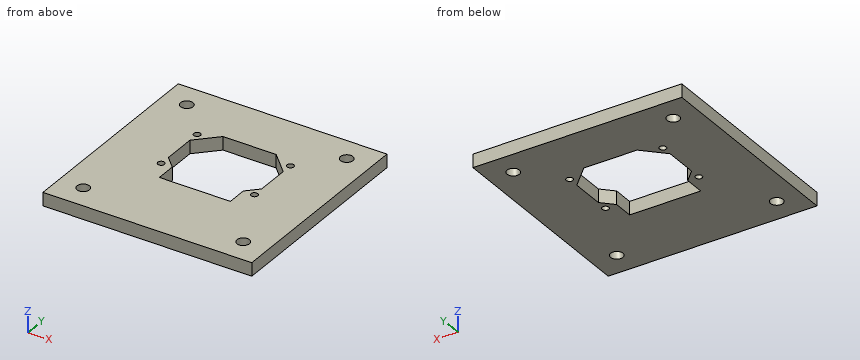
Autodesk Inventor part; units mm, degrees
ref_plane "YZ Plane" through (0, 0, 0) normal (1, 0, 0) x (0, 1, 0)
ref_plane "XZ Plane" through (0, 0, 0) normal (0, 1, 0) x (-1, 0, 0)
ref_plane "XY Plane" through (0, 0, 0) normal (0, 0, 1) x (1, 0, 0)
sketch "Sketch1" plane through (0, 0, 0) normal (0, 0, 1) x (1, 0, 0)
  circle A0 centre (-10.5, 10) radius 0.75
  circle A1 centre (-10.5, -2.5) radius 0.75
  circle A2 centre (10.5, 10) radius 0.75
  circle A3 centre (10.5, -2.5) radius 0.75
  line L0 (6, 12) -> (10.5, 7.5)
  line L1 (10.5, 7.5) -> (10.5, 0)
  line L2 (0, 15.2771) -> (0, -20.9272) construction
  line L3 (10.5, 0) -> (8, -2.5)
  line L4 (8, -2.5) -> (8, -7)
  line L5 (-6, 12) -> (-10.5, 7.5)
  line L6 (-10.5, 7.5) -> (-10.5, 0)
  line L7 (-10.5, 0) -> (-8, -2.5)
  line L8 (-8, -2.5) -> (-8, -7)
  line L9 (8, -7) -> (-8, -7)
  line L10 (23.5, 23.5) -> (23.5, -23.5)
  line L11 (23.5, -23.5) -> (-23.5, -23.5)
  line L12 (-23.5, -23.5) -> (-23.5, 23.5)
  line L13 (-23.5, 23.5) -> (23.5, 23.5)
  line L14 (6, 12) -> (-6, 12)
  line L15 (12.5, 12.5) -> (12.5, -12.5) construction
  line L16 (-12.5, -12.5) -> (-12.5, 12.5) construction
  line L17 (12.5, -12.5) -> (23.5, -23.5) construction
  line L18 (12.5, 12.5) -> (23.5, 23.5) construction
  line L19 (-12.5, 12.5) -> (-23.5, 23.5) construction
  line L20 (-12.5, -12.5) -> (-23.5, -23.5) construction
  circle A4 centre (18, -18) radius 1.4
  circle A5 centre (18, 18) radius 1.4
  circle A6 centre (-18, 18) radius 1.4
  circle A7 centre (-18, -18) radius 1.4
  line L21 (12.5, 12.5) -> (-12.5, -12.5) construction
  line L22 (12.5, -12.5) -> (-12.5, 12.5) construction
  point P0 (0, 0)
  point P1 (0, 0)
  point P2 (0, 0)
  point P3 (-8.25, 9.75)
  point P4 (0, 0)
  point P5 (0, 0)
  dimension "d2" = 1.5
  dimension "d5" = 1.5
  dimension "d8" = 1.5
  dimension "d11" = 1.5
  dimension "d48" = 2.8
  dimension "d49" = 2.8
  dimension "d50" = 2.8
  dimension "d51" = 2.8
  dimension "d63" = 15.5564
  dimension "d64" = 7.7782
  dimension "d66" = 7.7782
  dimension "d67" = 7.7782
  dimension "d68" = 47
extrude "Extrusion1" add sketch "Sketch1" along normal blind 3
equation "\"d64\" = 0.5 * d63"
equation "\"d66\" = d64"
equation "\"d67\" = d64"
properties part number "Camera-Holder_Mount"
Build history of the part. All positions in model axes, mm. Coordinates: 2 decimals unless noted, no trailing zeros. Order: outer loops, then holes, each group sorted by start corner. A loop starts at its lowest first (then second) coordinate and runs counter-clockwise, first axis right, second up. Notation, with made-up numbers: (-16.5, 71) - (34.5, 71) arc R22 cw to (34.5, 94) - close; hole circle Ø2 at (50.25, 53). An arc over 180 degrees is marked (long way). Put each result on its own line as item: value.
1. Drop a flat-ended pin along its axis: P1, Ø0.9, axis at x = -10.5, y = -2.5, coming from the -Z side. Give the stop position or say it passes through.
Answer sheet:
P1: passes through
2. Saw through at A-A (y = -18). Write the cut outline in (x, z), and give its area (3 significant figures).
Answer sheet:
outline: (-23.5, 0) - (-19.4, 0) - (-19.4, 3) - (-23.5, 3) - close; (-16.6, 0) - (16.6, 0) - (16.6, 3) - (-16.6, 3) - close; (19.4, 0) - (23.5, 0) - (23.5, 3) - (19.4, 3) - close
area: 124 mm^2
3. Probe line 1 along Y through (x, z) = (18, 2.2); line 2 along Y through (x, z) = (4.5, 0.85); line 3 along X through (y, z) = (-18.5, 2). List the from-to ranges inside material, lowest first. Write a range as [from, to].
Answer sheet:
line 1: y = [-23.5, -19.4], [-16.6, 16.6], [19.4, 23.5]
line 2: y = [-23.5, -7], [12, 23.5]
line 3: x = [-23.5, -19.31], [-16.69, 16.69], [19.31, 23.5]
4. Saw through at D-D (y = -4.5). Write the cut outline in (x, z).
Answer sheet:
outline: (-23.5, 0) - (-8, 0) - (-8, 3) - (-23.5, 3) - close; (8, 0) - (23.5, 0) - (23.5, 3) - (8, 3) - close
5. Saw through at C-C (x = 5). Write the cut outline in (y, z), and give its area (3 significant figures).
Answer sheet:
outline: (-23.5, 0) - (-7, 0) - (-7, 3) - (-23.5, 3) - close; (12, 0) - (23.5, 0) - (23.5, 3) - (12, 3) - close
area: 84.0 mm^2
